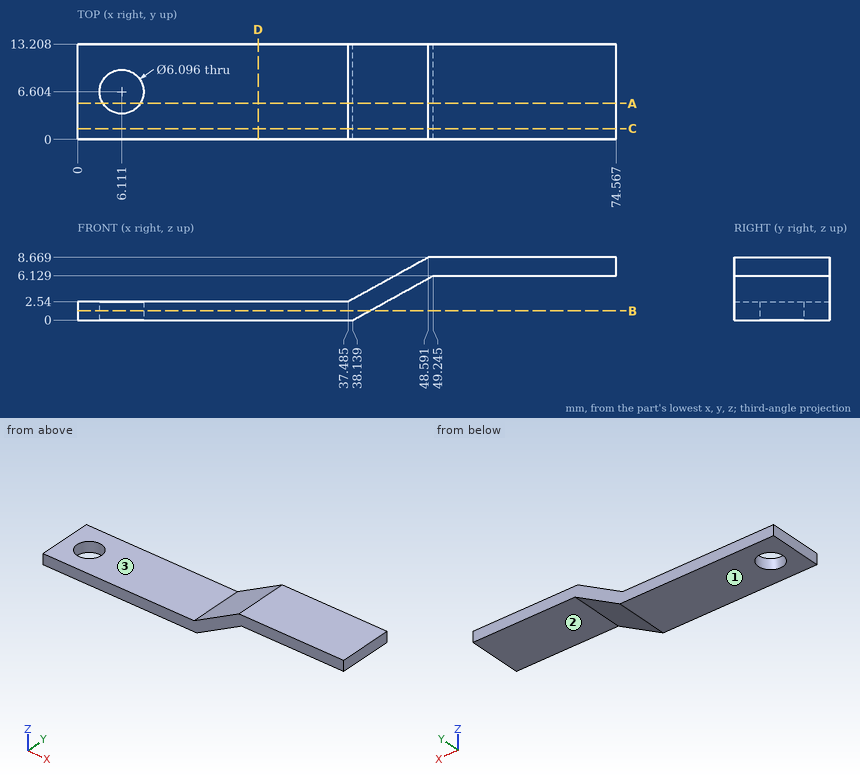
For this review, use the dimensioned drawing (mm, ordinates from the lowest corner) and the shaded views. A direction names the side the tool comes from. Give positions to 0.01 mm unless a question says otherwise; leave off trailing zeros. Order: outer loops, then holes, each group sorted by start corner. A loop starts at its lowest first (then second) coordinate and runs counter-clockwise, first axis right, second up.
1. For pin 1 Ø4 at (x, y) = (18.5, 8) entering from +Z; pin 2 Ø1.5 at (x, y) = (33, 7.5) entering from -Z; pin 3 Ø1 at (y, z) = (6, 4.5) entering from +X; pin 4 Ø6.5 at (x, y) = (62.5, 6.5) entering from -Z, all flat-tipped, find the tip position at first contact; note any pin that passes through.
Solution:
pin 1: stops at z = 2.54
pin 2: stops at z = 0
pin 3: stops at x = 47.2
pin 4: stops at z = 6.13
2. Add section C-C, the plane y = 1.5. State the section outline as (x, z) points (1 decimal).
Solution:
outline: (0, 0) - (38.1, 0) - (49.2, 6.1) - (74.6, 6.1) - (74.6, 8.7) - (48.6, 8.7) - (37.5, 2.5) - (0, 2.5) - close
3. To check wall thickness, follow L1, parallel to Z at x = 55, y = 10.5; L2, parallel to Z at x = 27, y = 12.25; L3, parallel to X at y = 8, z = 1.75 (1 decimal). State the ranges of each line that lie inside material, in increasing order.
Solution:
L1: z = 6.13 to 8.67
L2: z = 0 to 2.54
L3: x = 0 to 3.4, 8.8 to 41.3
4. Add section B-B, the plane z = 1.25. State the section outline as (x, y) points (1 decimal).
Solution:
outline: (0, 0) - (40.4, 0) - (40.4, 13.2) - (0, 13.2) - close; hole circle Ø6.1 at (6.1, 6.6)
5. Tool access review of the marked faces 1, 2 and 3: name each direction out of +Z, -Z, +X, -X, +Y, -Y from which nothing blocks a thin tool from reaching the whole face with its end or side.
Solution:
face 1: -Z, +X, -X, +Y, -Y
face 2: -Z, +X, +Y, -Y
face 3: +Z, -X, +Y, -Y
6. Add section A-A, the plane y = 5. State the section outline as (x, z) points (1 decimal), then the cut area to 3 significant figures.
Solution:
outline: (0, 0) - (3.5, 0) - (3.5, 2.5) - (0, 2.5) - close; (8.7, 0) - (38.1, 0) - (49.2, 6.1) - (74.6, 6.1) - (74.6, 8.7) - (48.6, 8.7) - (37.5, 2.5) - (8.7, 2.5) - close
area: 180 mm2
7. Add section D-D, the plane x = 25. State the section outline as (y, z) points.
Solution:
outline: (0, 0) - (13.21, 0) - (13.21, 2.54) - (0, 2.54) - close
